Input: part model. Units: mm. Frame: model coordinates. A direction names the side the tool comes from. Coordinates: 2 decimals unless noted, no trailing zeros. Loops run counter-clockwise (first coordinate to the right, second up) from the corner with the lowest first, then second, coordinate; pieces in that order, holes last. Notation, with made-up numbers: M 78.5,19 L 95.5,19 A35 ccw 95.5,55 Z; hole C 46.25,-7 d7. An arc over 180 degrees is marked long. Use a Markdown table: item, result. Add a question column.
1. Set-up query: faces 4 (the flat face through (-33, 15, 55)), 5 (the cylindrical face through (1.97, 7.4, -14.19)). Return all of +Z, -Z, +X, -X, +Y, -Y with unobstructed straight access to the full face (end or side cutting, diameter ignored); none if empty.
2. Section C-C on z = 54.5. Output: boundary loops of the cut face in (x, y), then the cut area to 3 significant figures.
3. Section B-B on y = 4.25. Output: boundary loops of the cut face in (x, z).
4. Section A-A on x = -5.5. Output: boundary loops of the cut face in (y, z), then the cut area to 3 significant figures.
5. Line query: L1, parallel to X at y = 4.5, z = 94; L2, parallel to X at y = 4, z = 43.5; L3, parallel to Z at x = -13, y = 12. Output: solid intervals per line, ascending. Write a range as [from, to].
6. Pin query (flat end, axial travel): pin 1 (10 mm diameter, centred on x = -33.5, z = 29, fed in from +Y); pin 2 (3 mm diameter, centred on y = 10.5, z = 96, fed in from -X); pin 3 (5 mm diameter, centred on x = -21.5, y = 12.5, fed in from +Z); pin 4 (3 mm diameter, centred on x = -3, y = 5, fed in from +Z). Return the tip coordinate at first contact, or that it passes through.
7. Draft query along Z for faces 1 (the cylindrical face through (-18.91, 7.4, 123.11)), 2 (the flat face through (-30.24, 7.4, 39.44)), 3 (the flat face through (-33, 0, 55)). Return one class per face: +Z half, -Z half, draft (parallel to the pull), parting line (faces both ways), or undercut.
Autodesk Inventor part; units mm, degrees
ref_plane "YZ Plane" through (0, 0, 0) normal (1, 0, 0) x (0, 1, 0)
ref_plane "XZ Plane" through (0, 0, 0) normal (0, 1, 0) x (-1, 0, 0)
ref_plane "XY Plane" through (0, 0, 0) normal (0, 0, 1) x (1, 0, 0)
sketch "Sketch1" plane through (0, 0, 0) normal (0, 1, 0) x (-1, 0, 0)
  circle A0 centre (0, 0) radius 14.3256 construction
  circle A1 centre (15.0854, 94.7166) radius 28.6512 construction
  line L0 (15.0854, 94.7166) -> (0, 0) construction
  line L1 (0, 0) -> (0, 94.7166) construction
  line L2 (0, 94.7166) -> (15.0854, 94.7166) construction
  line L3 (42.3895, 86.0345) -> (13.652, -4.3411)
  line L4 (-13.5648, 94.9463) -> (-14.3251, 0.1149)
  arc A2 (42.3895, 86.0345) -> (-13.5648, 94.9463) centre (15.0854, 94.7166) ccw
  arc A3 (-14.3251, 0.1149) -> (13.652, -4.3411) centre (0, 0) ccw
  arc A4 (-16.8651, 0.1352) -> (16.0726, -5.1107) centre (0, 0) ccw
  line L5 (16.0726, -5.1107) -> (44.8101, 85.2648)
  arc A5 (44.8101, 85.2648) -> (-16.1048, 94.9667) centre (15.0854, 94.7166) ccw
  line L6 (-16.1048, 94.9667) -> (-16.8651, 0.1352)
  point P0 (-16.8651, 0.1352)
  point P1 (-14.3251, 0.1149)
  dimension "d0" = 28.6512
  dimension "d1" = 57.3024
  dimension "d2" = 95.9104
  dimension "d3" = 94.7166
  dimension "d4" = 2.54
extrude "Extrusion1" add sketch "Sketch1" along normal blind 15
equation "\"d1\" = 2 * d0"
properties part number "ELEV_028_BELT1" material "Rubber"
Answers below:
| question | item | result |
|---|---|---|
| 1 | face 4 | +Z, -Z, +X, -X, +Y |
| 1 | face 5 | +Y, -Y |
| 2 | outline | M -35.03,0 L -32.36,0 L -32.36,15 L -35.03,15 Z; M 13.89,0 L 16.43,0 L 16.43,15 L 13.89,15 Z |
| 2 | area | 78.1 mm² |
| 3 | outline | M -44.81,85.26 L -16.07,-5.11 A16.87 ccw 16.87,0.14 L 16.1,94.97 A31.19 ccw long Z; hole M -42.39,86.03 L -13.65,-4.34 A14.33 ccw 14.33,0.11 L 13.56,94.95 A28.65 ccw long Z |
| 4 | outline | M 0,-15.94 L 15,-15.94 L 15,-13.23 L 0,-13.23 Z; M 0,121.72 L 15,121.72 L 15,124.4 L 0,124.4 Z |
| 4 | area | 81.0 mm² |
| 5 | L1 | x = [-46.27, -43.73], [13.57, 16.11] |
| 5 | L2 | x = [-31.53, -28.86], [13.98, 16.52] |
| 5 | L3 | z = [-10.74, -6.02], [123.29, 125.84] |
| 6 | pin 1 | passes through |
| 6 | pin 2 | stops at x = -46.28 |
| 6 | pin 3 | stops at z = 125.66 |
| 6 | pin 4 | stops at z = 124.06 |
| 7 | face 1 | undercut |
| 7 | face 2 | -Z half |
| 7 | face 3 | draft |
